Autodesk Inventor part; units mm, degrees
ref_plane "YZ Plane" through (0, 0, 0) normal (1, 0, 0) x (0, 1, 0)
ref_plane "XZ Plane" through (0, 0, 0) normal (0, 1, 0) x (-1, 0, 0)
ref_plane "XY Plane" through (0, 0, 0) normal (0, 0, 1) x (1, 0, 0)
sketch "Sketch1" plane through (0, 0, 0) normal (0, 0, 1) x (1, 0, 0)
  line L0 (0, -69) -> (57, -69)
  line L1 (57, -69) -> (57, 0)
  line L2 (57, 0) -> (117, 0)
  line L3 (117, 0) -> (117, 10)
  line L4 (117, 10) -> (57, 10)
  line L5 (57, 10) -> (57, 298)
  line L6 (57, 298) -> (0, 298)
  line L7 (0, 298) -> (0, -69) construction
  line L8 (0, -69) -> (-57, -69)
  line L9 (-57, -69) -> (-57, 0)
  line L10 (-57, 0) -> (-117, 0)
  line L11 (-117, 0) -> (-117, 10)
  line L12 (-117, 10) -> (-57, 10)
  line L13 (-57, 10) -> (-57, 298)
  line L14 (-57, 298) -> (0, 298)
  point P0 (0, 0)
  dimension "d0" = 57
  dimension "d2" = 10
  dimension "d18" = 367
  dimension "d19" = 117
  dimension "d47" = 69
extrude "Extrusion1" add sketch "Sketch1" along normal blind 83
sketch "Sketch2" plane through (0, 0, 0) normal (0, 0, -1) x (-1, 0, 0)
  line L0 (57, -69) -> (-57, -69)
  line L1 (57, 0) -> (57, -69)
  line L2 (117, 0) -> (57, 0)
  line L3 (117, 10) -> (117, 0)
  line L4 (57, 10) -> (117, 10)
  line L5 (57, 298) -> (57, 10)
  line L6 (-57, 298) -> (57, 298)
  line L7 (-57, 10) -> (-57, 298)
  line L8 (-117, 10) -> (-57, 10)
  line L9 (-117, 0) -> (-117, 10)
  line L10 (-57, 0) -> (-117, 0)
  line L11 (-57, -69) -> (-57, 0)
  point P0 (0, 0)
extrude "Extrusion2" add sketch "Sketch2" along normal blind 60
sketch "Sketch3" plane through (-57, 298, 83) normal (0, 1, 0) x (1, 0, 0)
  circle A0 centre (57, 82) radius 10
  line L0 (0, 143) -> (114, 143)
  line L1 (57, 82) -> (57, 143) construction
  dimension "d10" = 20
  dimension "d51" = 61
extrude "Extrusion3" cut sketch "Sketch3" against normal blind 10
sketch "Sketch4" plane through (-117, 10, 83) normal (0, 1, 0) x (1, 0, 0)
  line L0 (0, 143) -> (60, 143)
  line L1 (0, 143) -> (0, 0)
  line L2 (21.34, 84) -> (21.34, 143)
  line L3 (118.34, 120.2658) -> (118.34, -20.3509) construction
  line L4 (21.34, 84) -> (118.34, 84) construction
  circle A0 centre (21.34, 84) radius 10
  point P0 (117, 83)
  dimension "d21" = 59
  dimension "d23" = 97
  dimension "d24" = 20
extrude "Extrusion4" cut sketch "Sketch4" against normal through all
mirror "Mirror1" about plane through (0, 0, 0) normal (1, 0, 0) of "Extrusion4"
sketch "Sketch5" plane through (57, 10, 83) normal (0, 1, 0) x (1, 0, 0)
  line L0 (0, 143) -> (0, 0)
  line L1 (60, 143) -> (60, 0)
  line L2 (60, 143) -> (0, 143)
  line L3 (0, 143) -> (0, 105.1637)
  line L4 (0, 105.1637) -> (60, 105.1637)
  line L5 (60, 105.1637) -> (60, 143)
  line L6 (0, 0) -> (60, 0)
  line L7 (60, 0) -> (60, 62.9414)
  line L8 (60, 62.9414) -> (0, 62.9414)
  line L9 (0, 62.9414) -> (0, 0)
  point P0 (-57, 83)
extrude "Extrusion5" cut sketch "Sketch5" against normal through all contours L2 L1 L4 L0 | L8 L1 L6 L0
mirror "Mirror2" about plane through (0, 0, 0) normal (1, 0, 0) of "Extrusion5"
sketch "Sketch6" plane through (57, 10, -22.1637) normal (0, 1, 0) x (1, 0, 0)
  circle A0 centre (38.66, -21.1637) radius 10
  circle A1 centre (38.66, -21.1637) radius 19.7186
  point P0 (-57, -22.1637)
extrude "Extrusion6" add sketch "Sketch6" along normal blind 114 contours A0 | A1
mirror "Mirror3" about plane through (0, 0, 0) normal (1, 0, 0) of "Extrusion6"
move or copy body "Move Body3" bodies to move or copy 1 copy no rotation origin (0, 0, 0) rotation axis (0, 1, 0) rotation angle 90
move or copy body "Move Body4" bodies to move or copy 1 copy no rotation origin (0, 0, 0) rotation axis (1, 0, 0) rotation angle 90
move or copy body "Move Body8" bodies to move or copy 1 copy no translate (0, 0, 75)
properties part number "LowerTorso_v2"
Read the model definition and answer for the solid it produces. Units are mm, in the model's axes. A direction names the side the tool comes from. Coordinates: 2 decimals unless noted, no trailing zeros. Write each loop counter-clockwise with the first axis right and the second up, starting at its lowest first coordinate (ties: lowest second). Pieces come first, ordered by that corner, then holes. Notation, with made-up numbers: M 43,37 L 81,37 A24 cw 81,58 Z; hole C 53.25,-13 d7. An arc over 180 degrees is marked long. Use a Markdown table: item, result.
Q1. Each of these flat-tipped pins is pushed along its axis until it touches: pin 1 Ø6 at (x, y) = (-0.5, 93.5) entering from -Z; pin 2 Ø12 at (y, z) = (88, 79) entering from +X; pin 3 Ø16 at (x, y) = (-2, -92.5) entering from -Z. Where does it stop, or does it pass through?
Answer block:
| item | result |
|---|---|
| pin 1 | stops at z = 85 |
| pin 2 | stops at x = 20.06 |
| pin 3 | stops at z = 75 |
Q2. Which of the six approach directions +Z, -Z, +X, -X, +Y, -Y give full straight-line access (tool end or side, diameter ignored) to faces 4 (the face through (2.83, -86.423, 80.07)), 5 (the face through (10.76, -2.17, 368.07)), 6 (the face through (-6, 86.6, 75)), 7 (the face through (-6, -86.6, 75))?
Answer block:
| item | result |
|---|---|
| face 4 | -Z |
| face 5 | +Z |
| face 6 | -Z, +X, -X, +Y |
| face 7 | -Z, +X, -X, -Y |
Q3. Straight lines are drawn through the part: L1, parallel to X at y = -95, z = 82; L2, parallel to Y at x = 1, z = 371; L3, parallel to X at y = 0, z = 370. For each, find the intervals that lie inside material, in ascending order. Write a range as [from, to].
Answer block:
| item | result |
|---|---|
| L1 | x = [-22.16, -10.98], [8.98, 20.06] |
| L2 | y = [-57, -10], [10, 57] |
| L3 | x = [-60, -9], [11, 83] |
Q4. The part is cut by section A-A, the plane y = 95.66. Write down the section's boundary in (x, z), then the cut area to 3 significant figures.
Answer block:
| item | result |
|---|---|
| outline | M -22.16,75 L -11,75 L -11,85 L 9,85 L 9,75 L 20.06,75 L 20.06,85 L 18.72,85 L 18.72,199 L -20.72,199 L -20.72,85 L -22.16,85 Z |
| area | 4,720 mm2 |
Q5. The part is cut by section C-C, the plane z = 309. Write down the section's boundary in (x, y).
Answer block:
| item | result |
|---|---|
| outline | M -60,-57 L 83,-57 L 83,57 L -60,57 Z |
Q6. Determine the mould class of faces 1 (the face through (-60, 1, 192)), 2 (the face through (-1, -96, 85)), 3 (the face through (-1, -117, 80)) for opening direction Y: released by +Y, released by -Y, zero draft, split by the parting line, or undercut.
Answer block:
| item | result |
|---|---|
| face 1 | zero draft |
| face 2 | undercut |
| face 3 | released by -Y |
Q7. The part is cut by section B-B, the plane x = 49.5. Write down the section's boundary in (y, z), then the cut area to 3 significant figures.
Answer block:
| item | result |
|---|---|
| outline | M -57,6 L 57,6 L 57,373 L -57,373 Z |
| area | 41,800 mm2 |
